For this review, take the finished solid that the model builds, in its own axes (mm). A direction names the side the tool comes from. Give positions to 0.01 mm unless a question says otherwise; leave off trailing zeros. Order: outer loops, then holes, each group sorted by start corner. A loop starts at its lowest first (then second) coordinate and runs counter-clockwise, first axis right, second up. Notation, with made-up numbers: (-15, 46.25) - (17, 46.25) arc R22 cw to (17, 74.25) - close; hole circle Ø11 at (31, 42). An arc over 180 degrees is marked (long way). One line per item, written item: value.
```python
from build123d import *

# Parameters (mm, degrees)
F0_W      = 11.0998
F0_H      = 1.5748
F1_DEPTH  = 12.7
F3_DEPTH  = 9.525
F5_DEPTH  = 6.35
F6_SIZE2  = 10.998513
F6_SIZE   = 6.34999
F7_SIZE   = 3.17499
F8_SIZE   = 2.54
F9_W      = 15.0514596415
F9_H      = 12.7
F10_DEPTH = 25.4
F11_DEPTH = 76.2
F13_DEPTH = 25.4
F15_DEPTH = 25.4
F16_R     = 2.54


# Not quite as in the source:
# - a fillet or chamfer is up to 0.001 mm smaller than in the source, because OpenCascade refuses the exact size


with BuildPart() as f1:
    # F0 (on Top) → F1 (new body)
    with BuildSketch(Plane.XY):
        Polygon((19.0723874551, 12.7), (-4.7528125449, 12.7), (-4.7528125449, 1.5748), (-4.7528125449, 0), (19.0723874551, 0), align=None)
        Polygon((-15.8526125449, 12.7), (-19.0276125449, 12.7), (-19.0276125449, 0), (-15.8526125449, 0), (-15.8526125449, 1.5748), align=None)
        with Locations((-10.3027125449, 0.7874)):
            Rectangle(F0_W, F0_H)
    extrude(amount=F1_DEPTH)

    # F2 (on face) → F3 (cut)
    with BuildSketch(Plane(origin=(0, 0, 0), x_dir=(1, 0, 0), z_dir=(0, 0, -1))):
        Polygon((1.5971874551, -12.7), (1.5971874551, -1.5748), (1.5971874551, 0), (-19.0276125449, 0), (-19.0276125449, -12.7), align=None)
    extrude(amount=-F3_DEPTH, mode=Mode.SUBTRACT)

    # F4 (on face) → F5 (join)
    with BuildSketch(Plane.XY.offset(12.7)):
        Polygon((-15.8526125449, 12.7), (-19.0276125449, 12.7), (-19.0276125449, 0), (-4.7528125449, 0), (-4.7528125449, 1.5748), (-15.8526125449, 1.5748), align=None)
    extrude(amount=F5_DEPTH)

    # F6 (size 6.35 and 10.9985226281 in the source; OpenCascade refuses exactly that, so slightly less here)
    f6_edges = [f1.edges().sort_by_distance(p)[0] for p in [
        (-4.752813, 0.7874, 19.05),
    ]]
    f6_side = f1.faces().sort_by_distance((-4.752813, 0.7874, 15.875))[0]
    chamfer(f6_edges, length=F6_SIZE, length2=F6_SIZE2, reference=f6_side)

    # F7 (size 3.175 in the source; OpenCascade refuses exactly that, so slightly less here)
    f7_edges = [f1.edges().sort_by_distance(p)[0] for p in [
        (-4.752813, 7.1374, 12.7),
    ]]
    chamfer(f7_edges, length=F7_SIZE)

    # F8
    f8_edges = [f1.edges().sort_by_distance(p)[0] for p in [
        (19.072387, 6.35, 12.7),
        (19.072387, 6.35, 0),
        (19.072387, 12.7, 6.35),
    ]]
    chamfer(f8_edges, length=F8_SIZE)

    # F9 (on face) → F10 (cut)
    with BuildSketch(Plane.XY.offset(12.7)):
        with Locations((15.0030172759, 6.35)):
            Rectangle(F9_W, F9_H)
    extrude(amount=-F10_DEPTH, mode=Mode.SUBTRACT)

    # F11 (add): a face of the model
    f11_faces = [f1.faces().sort_by_distance(p)[0] for p in [
        (7.4772874551, 6.35, 6.35),
    ]]
    extrude(f11_faces, amount=F11_DEPTH)

    # F12 (on face) → F13 (cut)
    with BuildSketch(Plane(origin=(0, 12.7, 0), x_dir=(-1, 0, 0), z_dir=(0, 1, 0))):
        with BuildLine():
            Line((-23.4008067042, 0), (-4.3508067042, 0))
            ThreePointArc((-4.3508067042, 0), (-13.8758067042, 9.525), (-23.4008067042, 0))
        make_face()
    extrude(amount=-F13_DEPTH, mode=Mode.SUBTRACT)

    # F14 (on face) → F15 (cut)
    with BuildSketch(Plane(origin=(0, 12.7, 0), x_dir=(-1, 0, 0), z_dir=(0, 1, 0))):
        Polygon((-83.6772874551, 0), (-28.7684481591, 0), (-83.6772874551, 6.35), align=None)
    extrude(amount=-F15_DEPTH, mode=Mode.SUBTRACT)

    # F16
    f16_edges = [f1.edges().sort_by_distance(p)[0] for p in [
        (83.677287, 6.35, 12.7),
        (83.677287, 6.35, 6.35),
    ]]
    fillet(f16_edges, radius=F16_R)


solid = f1.part
```
(1) Take a section at D-D (z = 11.75). Write out the cut boundary in (x, y), then the cut area to 3 significant figures.
Answers below:
outline: (-19.03, 0) - (83.12, 0) - (83.12, 12.7) - (-2.53, 12.7) - (-2.53, 1.57) - (-15.85, 1.57) - (-15.85, 12.7) - (-19.03, 12.7) - close
area: 1,150 mm^2
(2) Draft analysis for pull direction X (two halves, no side actions). For faces 1 (the face through (-3.19, 7.22, 11.09)), 2 (the face through (1.597, 6, 5)), 3 (the face through (-4, 6, 9.525)), 4 (the face through (-10.33, 0.78, 15.92)), state which applies: pulls with the +X half, pulls with the -X half, needs draft (parallel to the pull), parting line crosses it, or undercut.
Answers below:
face 1: undercut
face 2: pulls with the -X half
face 3: needs draft
face 4: pulls with the +X half
(3) Take a section at B-B (z = 4). Write out the cut boundary in (x, y).
Answers below:
outline: (1.6, 0) - (5.23, 0) - (5.23, 12.7) - (1.6, 12.7) - close; (22.52, 0) - (63.36, 0) - (63.36, 12.7) - (22.52, 12.7) - close
(4) For P1, Ø7.5, axis at x = -9.5, z = 13.5, coming from the +Y side; P2, Ø1.5, axis at x = 15.5, z = 7, coming from the +Y side; P3, Ø4, axis at x = 38.5, y = 7, coming from the +Z side; P4, Ø6.5, axis at x = -13.5, y = 3.5, coming from the -Z side (3 decimals), all flat-tipped, find the tip position at first contact; note any pin that passes through.
Answers below:
P1: stops at y = 1.57
P2: passes through
P3: stops at z = 12.7
P4: stops at z = 9.525
(5) Wall thickness on line 1 (X direction, y = 8.25, z = 18); line 2 (Z direction, x = 2.5, y = 2.5); line 3 (Z direction, x = 14, y = 7.25): over which ranges is each line inside the solid? List them lowest first. Write a range as from..to.
Answers below:
line 1: x = -19.03..-15.85
line 2: z = 0..12.7
line 3: z = 9.52..12.7
(6) Machinability: for faces 5 (the face through (-15.853, 7, 14)), 6 (the face through (54.7, 6.4, 3)), 7 (the face through (38, 6, 12.7)), which of the approach directions +Z, -Z, +X, -X, +Y, -Y give a long, thin tool a straight path to every point of the face, cutting with its end or side? Answer none if there is none.
Answers below:
face 5: +Z, -Z, +Y
face 6: -Z, +X, +Y, -Y
face 7: +Z, +X, +Y, -Y
(7) Take a section at C-C (x = 49.5). Write out the cut boundary in (y, z).
Answers below:
outline: (0, 2.4) - (12.7, 2.4) - (12.7, 12.7) - (0, 12.7) - close
